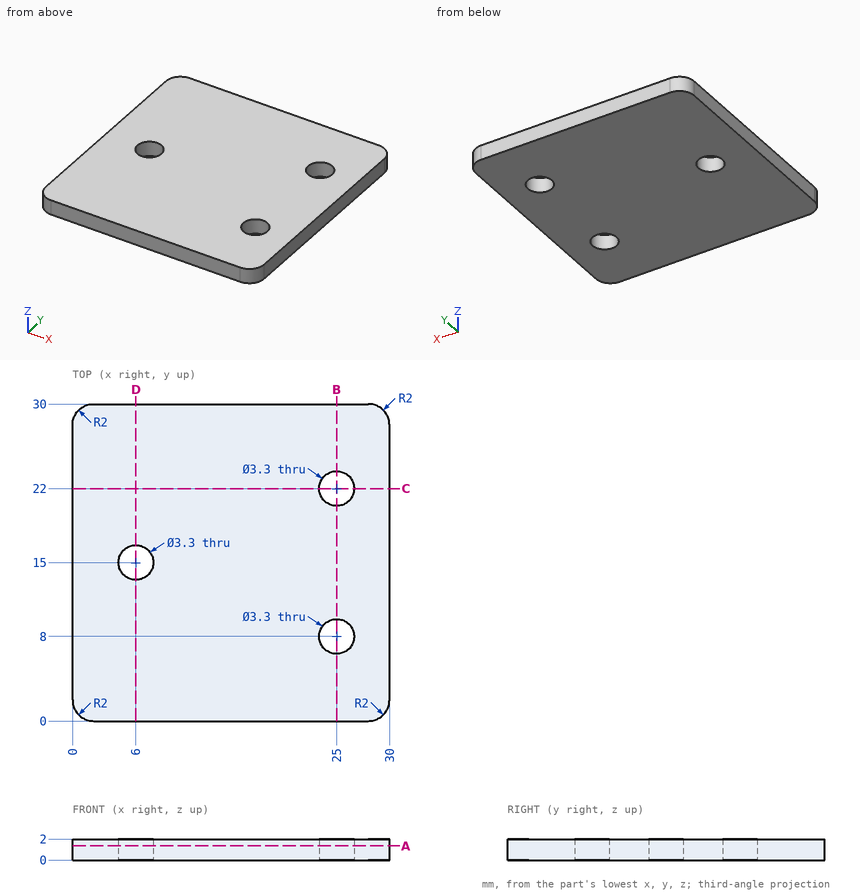
Part print with two shaded views. Sizes in mm from the minimum x, y, z corner. Coordinates: 2 decimals unless noted, no trailing zeros. Write each loop counter-clockwise with the first axis right and the second up, starting at its lowest first coordinate (ties: lowest second). Pieces come first, ordered by that corner, then holes. Notation, with made-up numbers: (-2, -12) - (20, -12) arc R27 ccw to (20, 27) - close; hole circle Ø5 at (73, -31.75). An arc over 180 degrees is marked (long way). Put each result on its own line as item: value.
1. Band-saw the part on B-B (x = 25). Write the cut outline in (y, z), then the cut area to 3 significant figures.
Final values:
outline: (0, 0) - (6.35, 0) - (6.35, 2) - (0, 2) - close; (9.65, 0) - (20.35, 0) - (20.35, 2) - (9.65, 2) - close; (23.65, 0) - (30, 0) - (30, 2) - (23.65, 2) - close
area: 46.8 mm²
2. Band-saw the part on C-C (y = 22). Write the cut outline in (x, z), then the cut area to 3 significant figures.
Final values:
outline: (0, 0) - (23.35, 0) - (23.35, 2) - (0, 2) - close; (26.65, 0) - (30, 0) - (30, 2) - (26.65, 2) - close
area: 53.4 mm²
3. Band-saw the part on A-A (z = 1.35). Write the cut outline in (x, y), then the cut area to 3 significant figures.
Final values:
outline: (0, 2) arc R2 ccw to (2, 0) - (28, 0) arc R2 ccw to (30, 2) - (30, 28) arc R2 ccw to (28, 30) - (2, 30) arc R2 ccw to (0, 28) - close; hole circle Ø3.3 at (6, 15); hole circle Ø3.3 at (25, 8); hole circle Ø3.3 at (25, 22)
area: 871 mm²
4. Band-saw the part on D-D (x = 6). Write the cut outline in (y, z).
Final values:
outline: (0, 0) - (13.35, 0) - (13.35, 2) - (0, 2) - close; (16.65, 0) - (30, 0) - (30, 2) - (16.65, 2) - close
5. Flat gauge pin, fed straight in: pin 1 Ø2 at (x, y) = (25, 22) entering from +Z. Where does the tip first touch, or does it go through?
Final values:
pin 1: passes through
6. Probe line 1 along Y through (x, z) = (25, 1.4); line 2 along Y through (x, z) = (6, 1.95); line 3 along X through (y, z) = (7, 1.25). List the from-to ranges inside material, lowest first. Write a range as [from, to].
Final values:
line 1: y = [0, 6.35], [9.65, 20.35], [23.65, 30]
line 2: y = [0, 13.35], [16.65, 30]
line 3: x = [0, 23.69], [26.31, 30]
